Design review of the part shown in the three views and the two pictorial views. Dimensions are in mm from the part's minimum x, y and z. Give positions to 0.01 mm unless a question says otherwise; leave off trailing zeros. Order: outer loops, then holes, each group sorted by start corner. A loop starts at its lowest first (then second) coordinate and runs counter-clockwise, first axis right, second up. Notation, with made-up numbers: (38.5, 43.5) - (85.5, 43.5) arc R20 cw to (85.5, 77.5) - close; hole circle Ø3 at (12.25, -29). An arc over 180 degrees is marked (long way). Put each result on its own line as item: value.
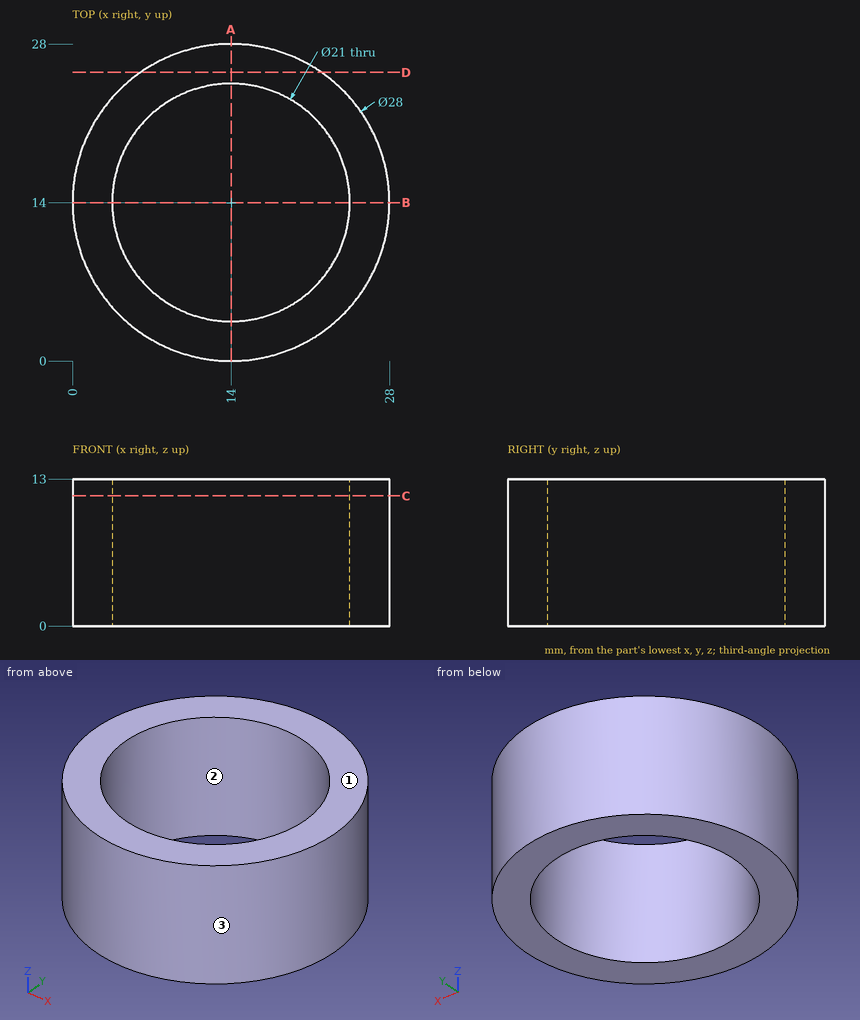
(1) Take a section at D-D, the plane y = 25.5. Write out the cut boundary in (x, z).
The answers:
outline: (6.02, 0) - (21.98, 0) - (21.98, 13) - (6.02, 13) - close
(2) Clearance check with flat-ended pins moving along their axes: pin 1 Ø8 at (x, y) = (18, 9) entering from -Z; pin 2 Ø3 at (y, z) = (11, 1.5) entering from +X; pin 3 Ø1 at (x, z) = (23.5, 9.5) entering from +Y; pin 4 Ø4 at (y, z) = (24.5, 8.5) entering from +X. State where each tip first meets the part, or that it passes through.
The answers:
pin 1: through
pin 2: x = 27.92
pin 3: y = 24.72
pin 4: x = 25.12
(3) The part is to be moulded in two halves that separate along Y. For the marked faces 1, 2 and 3, say which applies: pulls with the +Y half, pulls with the -Y half, needs draft (parallel to the pull), parting line crosses it, or undercut.
The answers:
face 1: needs draft
face 2: undercut
face 3: parting line crosses it
(4) Take a section at A-A, the plane x = 14. Write out the cut boundary in (y, z), then the cut area to 3 significant figures.
The answers:
outline: (0, 0) - (3.5, 0) - (3.5, 13) - (0, 13) - close; (24.5, 0) - (28, 0) - (28, 13) - (24.5, 13) - close
area: 91.0 mm^2
(5) Wall thickness on L1, parallel to Y at x = 14, z = 3.25; L2, parallel to X at y = 13.5, z = 9; L3, parallel to X at y = 21.5, z = 8.5: over which ranges is each line inside the solid? List them lowest first.
The answers:
L1: 0 to 3.5, 24.5 to 28
L2: 0.01 to 3.51, 24.49 to 27.99
L3: 2.18 to 6.65, 21.35 to 25.82
(6) Take a section at C-C, the plane z = 11.5. Write out the cut boundary in (x, y), then the cut area to 3 significant figures.
The answers:
outline: circle Ø28 at (14, 14); hole circle Ø21 at (14, 14)
area: 269 mm^2
